```python
from build123d import *

# Parameters (mm, degrees)
F0_W     = 23.5
F0_H     = 23.5
F1_DEPTH = 11.75
F2_W     = 22
F2_H     = 22
F3_DEPTH = 50
F4_W     = 22
F4_H     = 22
F5_DEPTH = 50
F6_W     = 22
F6_H     = 22
F7_DEPTH = 50


with BuildPart() as f1:
    # F0 (on Front) → F1 (new body, symmetric)
    with BuildSketch(Plane.XZ):
        Rectangle(F0_W, F0_H)
    extrude(amount=F1_DEPTH, both=True)

    # F2 (on face) → F3 (join)
    with BuildSketch(Plane.XZ.offset(11.75)):
        Rectangle(F2_W, F2_H)
    extrude(amount=F3_DEPTH)

    # F4 (on face) → F5 (join)
    with BuildSketch(Plane.XY.offset(11.75)):
        Rectangle(F4_W, F4_H)
    extrude(amount=F5_DEPTH)

    # F6 (on face) → F7 (join)
    with BuildSketch(Plane.YZ.offset(11.75)):
        Rectangle(F6_W, F6_H)
    extrude(amount=F7_DEPTH)


solid = f1.part
```
Geometry check sheet. Reference: the model listing, model coordinates, mm. A direction names the side the tool comes from. Coordinates: 2 decimals unless noted, no trailing zeros. Loops run counter-clockwise (first coordinate to the right, second up) from the corner with the lowest first, then second, coordinate; pieces in that order, holes last. Notation, with made-up numbers: (46, 81.25) - (100, 81.25) arc R11 ccw to (100, 98.25) - close; hole circle Ø6 at (-4.75, 57). An arc over 180 degrees is marked (long way). One line per item, written item: value. Start each with the question number.
(1) Cross-section at C-C on y = -38.5. Enter the section's corners in (x, z), plus the area to 3 significant figures.
(2) Depth check by flat-ended pin: P1, Ø1.5, axis at y = -40.5, z = 1.5, coming from the -X side; P2, Ø5, axis at y = -37.5, z = 3.5, coming from the +X side; P3, Ø17.5, axis at x = 27.5, z = -3.5, coming from the +Y side. Enter the tip coordinate at first touch or a pass-through.
(3) Cross-section at A-A on x = -5.5. Enter the section's corners in (y, z).
(4) Material ranges on line 1 (Z direction, x = -4.5, y = -13.5), recorded low to high. Write a range as [from, to].
(5) Tool access check on faces 1 (the flat face through (0, -36, -11)), 2 (the flat face through (36, 0, -11)), 3 (the flat face through (0, 11, 36)), 4 (the flat face through (0, -36, 11)). Record the directions out of +Z, -Z, +X, -X, +Y, -Y that give a thin tool (end or side, any length) a straight path to the whole face; none if there is none.
(6) Cross-section at B-B on z = 8. Enter the section's corners in (x, y).
Results below:
1. outline: (-11, -11) - (11, -11) - (11, 11) - (-11, 11) - close
1. area: 484 mm2
2. P1: stops at x = -11
2. P2: stops at x = 11
2. P3: stops at y = 11
3. outline: (-61.75, -11) - (-11.75, -11) - (-11.75, -11.75) - (11.75, -11.75) - (11.75, 11.75) - (11, 11.75) - (11, 61.75) - (-11, 61.75) - (-11, 11.75) - (-11.75, 11.75) - (-11.75, 11) - (-61.75, 11) - close
4. line 1: z = [-11, 11]
5. face 1: -Z, +X, -X, -Y
5. face 2: -Z, +X, +Y, -Y
5. face 3: +Z, +X, -X, +Y
5. face 4: +Z, +X, -X, -Y
6. outline: (-11.75, -11.75) - (-11, -11.75) - (-11, -61.75) - (11, -61.75) - (11, -11.75) - (11.75, -11.75) - (11.75, -11) - (61.75, -11) - (61.75, 11) - (11.75, 11) - (11.75, 11.75) - (-11.75, 11.75) - close
